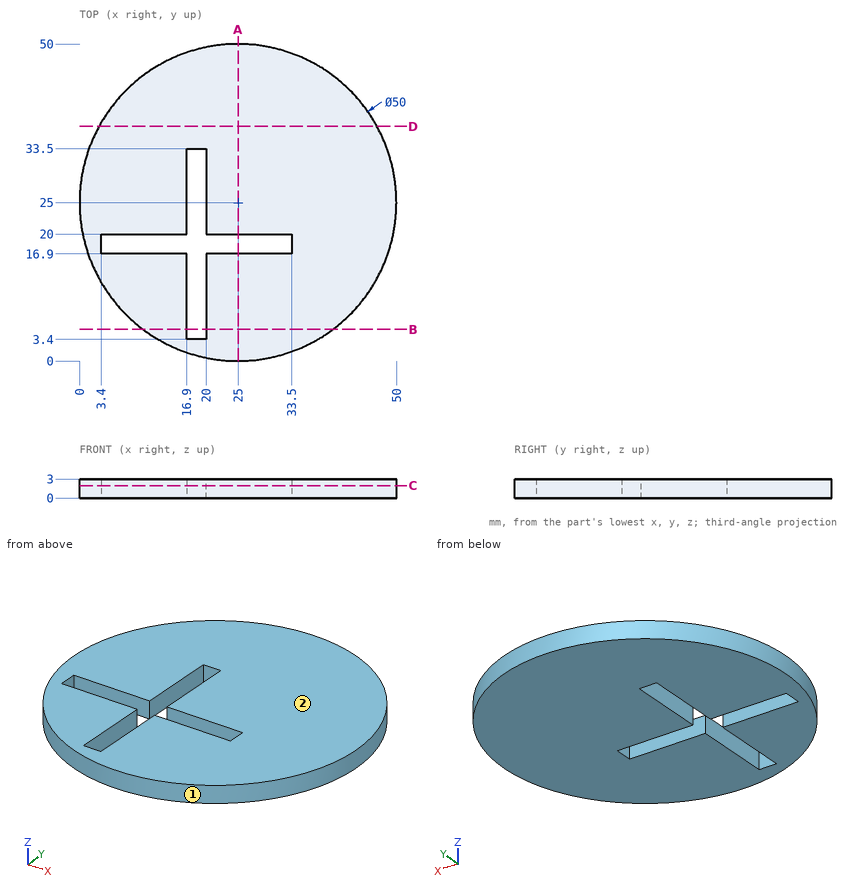
Source: three-view drawing plus pictorial views. Frame: mm from the lowest corner of the part. Give positions to 0.01 mm unless a question says otherwise; leave off trailing zeros. Write each loop counter-clockwise with the first axis right and the second up, starting at its lowest first coordinate (ties: lowest second). Pieces come first, ordered by that corner, then holes.
(1) Cut plane D-D, the plane y = 37. Return loops of the section in (x, z), then the cut area to 3 significant figures.
(2) Cut plane A-A, the plane x = 25. Return loops of the section in (y, z), then the cut area to 3 significant figures.
(3) Mould query, pull axis X, two halves, no side actions, for the marked faces 1 and 2. Classes: released by +X, released by -X, zero draft, split by the parting line, or undercut.
(4) First-contact query: P1, Ø1.5, axis at y = 18.5, z = 1, coming from the +X side; P2, Ø0.9, axis at x = 18, z = 1.5, coming from the -Y side; P3, Ø1.5, axis at x = 13, z = 1, coming from the +Y side. Flat tips, straight axial feed; report the tip coordinate or a pass-through.
(5) Ray query, line 1 (Y direction, x = 25, z = 1.65); line 2 (X direction, y = 24.5, z = 2.05) (3 decimals); line 3 (Y direction, x = 4, z = 0.3). Return the intervals inside material, ascending.
(6) Cut plane B-B, the plane y = 5. Return loops of the section in (x, z).
(7) Cut plane C-C, the plane z = 1.95. Return loops of the section in (x, y), then the cut area to 3 significant figures.
Values follow:
1. outline: (3.07, 0) - (46.93, 0) - (46.93, 3) - (3.07, 3) - close
1. area: 132 mm2
2. outline: (0, 0) - (16.9, 0) - (16.9, 3) - (0, 3) - close; (20, 0) - (50, 0) - (50, 3) - (20, 3) - close
2. area: 141 mm2
3. face 1: split by the parting line
3. face 2: zero draft
4. P1: stops at x = 49.33
4. P2: stops at y = 0.87
4. P3: stops at y = 47.33
5. line 1: y = 0 to 16.9, 20 to 50
5. line 2: x = 0.005 to 16.9, 20 to 49.995
5. line 3: y = 11.44 to 16.9, 20 to 38.56
6. outline: (10, 0) - (16.9, 0) - (16.9, 3) - (10, 3) - close; (20, 0) - (40, 0) - (40, 3) - (20, 3) - close
7. outline: circle Ø50 at (25, 25); hole (3.4, 16.9) - (16.9, 16.9) - (16.9, 3.4) - (20, 3.4) - (20, 16.9) - (33.5, 16.9) - (33.5, 20) - (20, 20) - (20, 33.5) - (16.9, 33.5) - (16.9, 20) - (3.4, 20) - close
7. area: 1,790 mm2
